```python
from build123d import *

# Parameters (mm, degrees)
SKETCH1_W           = 99
SKETCH1_H           = 6
BOSS_EXTRUDE1_DEPTH = 2
SKETCH2_W           = 101
SKETCH2_H           = 8
BOSS_EXTRUDE3_DEPTH = 2
DRAFT1_ANGLE        = 10
SKETCH3_W           = 103
SKETCH3_H           = 10
BOSS_EXTRUDE4_DEPTH = 2
FILLET1_R           = 2
CUT_EXTRUDE1_DEPTH  = 1


with BuildPart() as part:
    # Sketch1 → Boss-Extrude1 (new body)
    with BuildSketch(Plane(origin=(0, 0, 0), x_dir=(1, 0, 0), z_dir=(0, 1, 0))):
        Rectangle(SKETCH1_W, SKETCH1_H)
    extrude(amount=BOSS_EXTRUDE1_DEPTH)

    # Draft1
    draft1_faces = [part.faces().sort_by_distance(p)[0] for p in [
        (49.5, 1, 0),
        (0, 1, 3),
        (-49.5, 1, 0),
        (0, 1, -3),
    ]]
    draft(draft1_faces, Plane(origin=(0, 0, 0), x_dir=(0, 0, -1), z_dir=(0, -1, 0)), DRAFT1_ANGLE)



with BuildPart() as body_2:
    # Sketch2 → Boss-Extrude3 (new body)
    with BuildSketch(Plane(origin=(0, 2, 0), x_dir=(1, 0, 0), z_dir=(0, 1, 0))):
        Rectangle(SKETCH2_W, SKETCH2_H)
    extrude(amount=BOSS_EXTRUDE3_DEPTH)


with BuildPart() as part_1:
    add(part.part)

    add(body_2.part)  # Boss-Extrude4 merges body 2
    # Sketch3 → Boss-Extrude4 (add)
    with BuildSketch(Plane(origin=(0, 4, 0), x_dir=(1, 0, 0), z_dir=(0, 1, 0))):
        Rectangle(SKETCH3_W, SKETCH3_H)
    extrude(amount=-BOSS_EXTRUDE4_DEPTH)

    # Fillet1
    fillet1_edges = [part_1.edges().sort_by_distance(p)[0] for p in [
        (-51.5, 3, 5),
        (-51.5, 3, -5),
        (51.5, 3, -5),
        (51.5, 3, 5),
    ]]
    fillet(fillet1_edges, radius=FILLET1_R)

    # Sketch4 → Cut-Extrude1 (cut)
    with BuildSketch(Plane(origin=(0, 4, 0), x_dir=(1, 0, 0), z_dir=(0, 1, 0))):
        Polygon((-2.575148278, 1.834748189), (-2.238609816, 1.834748189), (-1.07194315, -0.923464952), (0.094723517, 1.834748189), (0.431261979, 1.834748189), (-1.049507252, -1.665251811), (-1.094379047, -1.665251811), align=None)
        Polygon((1.489254767, 1.834748189), (2.136390184, 1.834748189), (2.136390184, -1.665251811), (1.82228762, -1.665251811), (1.82228762, 1.47577383), (1.283826081, 1.47577383), align=None)
    extrude(amount=-CUT_EXTRUDE1_DEPTH, mode=Mode.SUBTRACT)


solid = part_1.part
```
For this review, take the finished solid that the model builds, in its own axes (mm). Coordinates: 2 decimals unless noted, no trailing zeros. Loops run counter-clockwise (first coordinate to the right, second up) from the corner with the lowest first, then second, coordinate; pieces in that order, holes last. Notation, with made-up numbers: (65, 62.5) - (99, 62.5) arc R22 cw to (99, 75.5) - close; hole circle Ø5 at (4.25, -39). An arc over 180 degrees is marked (long way). Use one line per item in the form item = value. Start each with the question number.
1) Draft analysis for pull direction X (two halves, no side actions). For faces 1 (the face through (49.674, 0.986, 0.047)), 2 (the face through (-1, 3, 5)), 3 (the face through (-51.5, 3, 0)), state which applies: released by +X, released by -X, zero draft, split by the parting line, or undercut.
2) Take a section at A-A (x = 28.5). State the section outline as (y, z) points, plus the area to 3 significant figures.
3) Take a section at B-B (y = 0.85). State the section outline as (x, z) points, plus the area to 3 significant figures.
4) To check wall thickness, follow probe 1 along Y at (x, z) = (-2.5, -4); probe 2 along Z at (x, y) = (1.5, 1.9); probe 3 along X at (y, z) = (2.75, -4.5). State the ranges of each line that lie inside material, in increasing order. Write a range as from..to.
From the geometry:
q1.face_1 = released by +X
q1.face_2 = zero draft
q1.face_3 = released by -X
q2.outline = (0, -3) - (2, -3.35) - (2, -5) - (4, -5) - (4, 5) - (2, 5) - (2, 3.35) - (0, 3) - close
q2.area = 32.7 mm2
q3.outline = (-49.65, -3.15) - (49.65, -3.15) - (49.65, 3.15) - (-49.65, 3.15) - close
q3.area = 626 mm2
q4.probe_1 = 2..4
q4.probe_2 = -3.34..3.34
q4.probe_3 = -50.82..50.82
